from build123d import *

# Parameters (mm, degrees)
F0_W     = 145
F0_H     = 95
F1_DEPTH = 25
F2_R     = 8
F3_W     = 135
F3_H     = 85
F4_DEPTH = 8
F5_R     = 8


with BuildPart() as f1:
    # F0 (on Top) → F1 (new body)
    with BuildSketch(Plane.XY):
        with Locations((-21.325343, 35.507629)):
            Rectangle(F0_W, F0_H)
    extrude(amount=F1_DEPTH)

    # F2
    f2_edges = [f1.edges().sort_by_distance(p)[0] for p in [
        (-93.825343, -11.992371, 12.5),
        (51.174657, -11.992371, 12.5),
        (51.174657, 83.007629, 12.5),
        (-93.825343, 83.007629, 12.5),
    ]]
    fillet(f2_edges, radius=F2_R)

    # F3 (on face) → F4 (cut)
    with BuildSketch(Plane.XY.offset(25)):
        with Locations((-21.325343, 35.507629)):
            Rectangle(F3_W, F3_H)
    extrude(amount=-F4_DEPTH, mode=Mode.SUBTRACT)

    # F5
    f5_edges = [f1.edges().sort_by_distance(p)[0] for p in [
        (-88.825343, 78.007629, 21),
        (-88.825343, -6.992371, 21),
        (46.174657, 78.007629, 21),
        (46.174657, -6.992371, 21),
    ]]
    fillet(f5_edges, radius=F5_R)


solid = f1.part
Geometry check sheet. Reference: the model listing, model coordinates, mm. A direction names the side the tool comes from. Round coordinates to 2 decimals unless told otherwise and drop trailing zeros. Loops run counter-clockwise (first coordinate to the right, second up) from the corner with the lowest first, then second, coordinate; pieces in that order, holes last. Notation, with made-up numbers: (-40, 63.5) - (-23, 63.5) arc R30 cw to (-23, 87.5) - close; hole circle Ø2 at (10, 27.25). An arc over 180 degrees is marked (long way). One line per question, with ' | ' between items. Start each with the question number.
1. Depth check by flat-ended pin: pin 1 (8 mm diameter, centred on x = -36, y = 16.5, fed in from +Z). Enter the tip coordinate at first touch or a pass-through.
2. Cross-section at B-B on x = -67.5. Record the cut outline in (y, z), then the cut area to 4 significant figures.
3. Cross-section at A-A on z = 18.5. Record the cut outline in (x, y).
4. Cross-section at C-C on y = 55.5. Record the cut outline in (x, z), then the cut area to 4 significant figures.
5. Tool access check on faces 4 (the face through (-22, 36, 17)), 5 (the face through (-22, -11.992, 12)). Record the directions out of +Z, -Z, +X, -X, +Y, -Y that give a thin tool (end or side, any length) a straight path to the whole face; none if there is none.
6. Scan lines: line 1 (Y direction, x = 19, z = 19.25); line 2 (X direction, y = 10, z = 18.25); line 3 (Z direction, x = -77, y = 2.5). Record each from-to range of solid material in increasing order. Write a range as [from, to].
7. Draft check along X on faces 1 (the face through (51.175, 35, 12)), 2 (the face through (-22, 36, 0)), 3 (the face through (-22, 78.008, 21)). Enter one of: released by +X, released by -X, zero draft, split by the parting line, or undercut.
Taken from the geometry:
1) pin 1: z = 17
2) outline: (-11.99, 0) - (83.01, 0) - (83.01, 25) - (78.01, 25) - (78.01, 17) - (-6.99, 17) - (-6.99, 25) - (-11.99, 25) - close | area: 1,695 mm²
3) outline: (-93.83, -3.99) arc R8 ccw to (-85.83, -11.99) - (43.17, -11.99) arc R8 ccw to (51.17, -3.99) - (51.17, 75.01) arc R8 ccw to (43.17, 83.01) - (-85.83, 83.01) arc R8 ccw to (-93.83, 75.01) - close; hole (-88.83, 1.01) arc R8 ccw to (-80.83, -6.99) - (38.17, -6.99) arc R8 ccw to (46.17, 1.01) - (46.17, 70.01) arc R8 ccw to (38.17, 78.01) - (-80.83, 78.01) arc R8 ccw to (-88.83, 70.01) - close
4) outline: (-93.83, 0) - (51.17, 0) - (51.17, 25) - (46.17, 25) - (46.17, 17) - (-88.83, 17) - (-88.83, 25) - (-93.83, 25) - close | area: 2,545 mm²
5) face 4: +Z | face 5: +Z, -Z, +X, -X, -Y
6) line 1: [-11.99, -6.99], [78.01, 83.01] | line 2: [-93.83, -88.83], [46.17, 51.17] | line 3: [0, 17]
7) face 1: released by +X | face 2: zero draft | face 3: undercut
